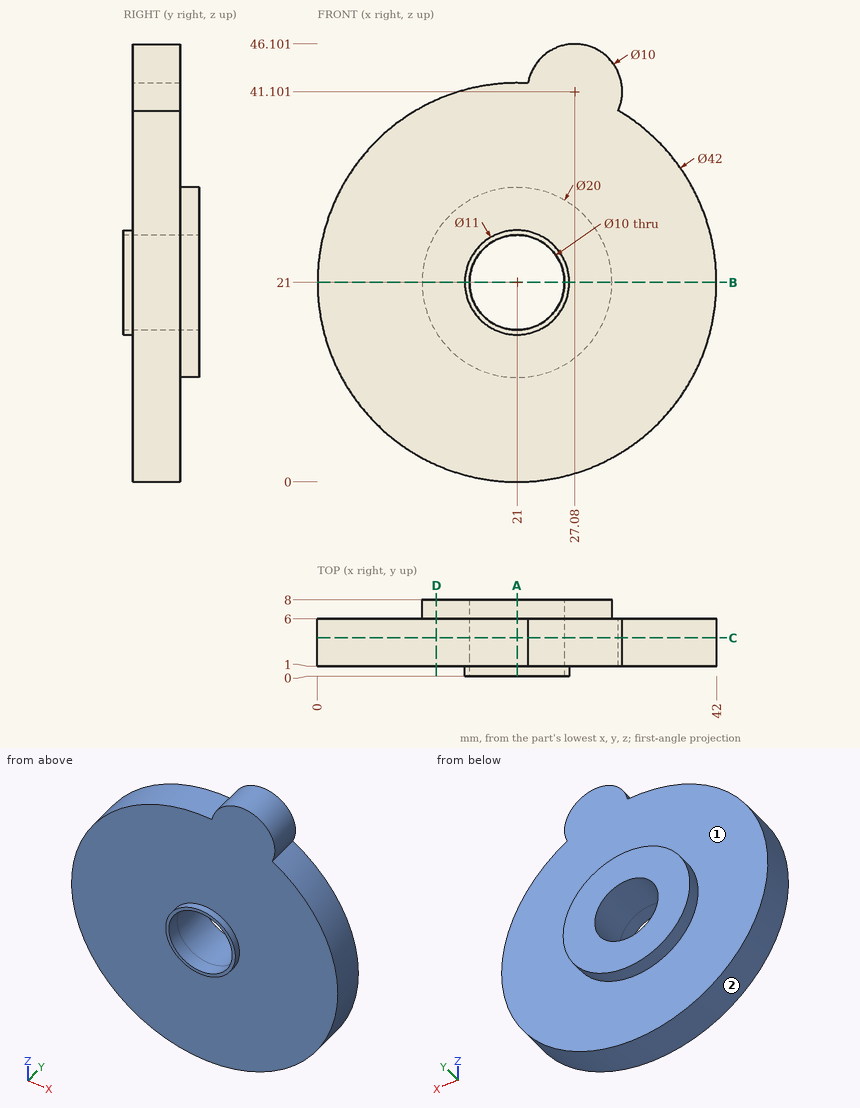
Drawing for the job (mm, zero at the part's lowest x, y, z). A direction names the side the tool comes from. Round coordinates to 2 decimals unless told otherwise and drop trailing zeros. Write each loop counter-clockwise with the first axis right and the second up, starting at its lowest first coordinate (ties: lowest second). Pieces come first, ordered by that corner, then holes. Notation, with made-up numbers: (56.25, 56) - (91.25, 56) arc R31 ccw to (91.25, 88) - close; hole circle Ø11 at (31.5, 32.25). An arc over 180 degrees is marked (long way). Use CSV: the item, a comma, the result in double quotes.
(1) Band-saw the part on B-B (z = 21). Write the cut outline in (x, y).
Response:
outline,"(0, 1) - (15.5, 1) - (15.5, 0) - (16, 0) - (16, 8) - (11, 8) - (11, 6) - (0, 6) - close; (26, 0) - (26.5, 0) - (26.5, 1) - (42, 1) - (42, 6) - (31, 6) - (31, 8) - (26, 8) - close"
(2) Pin check, flat tips, straight feed: P1, Ø2, axis at x = 23.5, y = 3.5, coming from the +Z side; P2, Ø2, axis at x = 7.5, z = 35.5, coming from the -Y side; P3, Ø1.5, axis at x = 6.5, y = 2.5, coming from the -Z side. Stop position of each tip, or through.
Response:
P1,"z = 45.38"
P2,"y = 1"
P3,"z = 5.13"
(3) Band-saw the part on D-D (x = 12.5). Write the cut outline in (y, z).
Response:
outline,"(1, 1.8) - (6, 1.8) - (6, 15.73) - (8, 15.73) - (8, 26.27) - (6, 26.27) - (6, 40.2) - (1, 40.2) - close"
(4) 3-axis set-ups, long thin cutter, end or side, ignore diameter. For the marked faces 1 and 2: which of +Z, -Z, +X, -X, +Y, -Y reach the whole face in a straight line?
Response:
face 1,"+Y"
face 2,"+Y, -Y"
(5) Band-saw the part on A-A (x = 21). Write the cut outline in (y, z).
Response:
outline,"(0, 15.5) - (1, 15.5) - (1, 0) - (6, 0) - (6, 11) - (8, 11) - (8, 16) - (0, 16) - close; (0, 26) - (8, 26) - (8, 31) - (6, 31) - (6, 42) - (1, 42) - (1, 26.5) - (0, 26.5) - close"
(6) Band-saw the part on C-C (y = 4). Write the cut outline in (x, z) (1 decimal), plus the area to 3 significant figures.
Response:
outline,"(22.2, 42) arc R21 ccw (long way) to (31.7, 39.1) arc R5 ccw (long way) to start; hole circle Ø10 at (21, 21)"
area,"1,350 mm²"
(7) Wall check: line 1 (Z direction, x = 21, y = 1.2); line 2 (Z direction, x = 21, y = 0.55); line 3 (Y direction, x = 7, z = 17). Give the ranges that are in metal, low to high.
Response:
line 1,"0 to 16, 26 to 42"
line 2,"15.5 to 16, 26 to 26.5"
line 3,"1 to 6"
